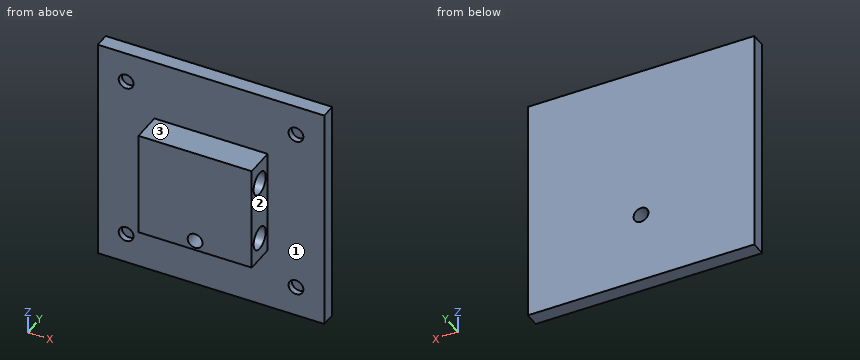
Autodesk Inventor part; units mm, degrees
ref_plane "YZ Plane" through (0, 0, 0) normal (1, 0, 0) x (0, 1, 0)
ref_plane "XZ Plane" through (0, 0, 0) normal (0, 1, 0) x (-1, 0, 0)
ref_plane "XY Plane" through (0, 0, 0) normal (0, 0, 1) x (1, 0, 0)
sketch "Sketch1" plane through (0, 0, 0) normal (1, 0, 0) x (0, 1, 0)
  line L0 (0, 0) -> (10, 0)
  line L1 (10, 0) -> (10, -20)
  line L2 (10, -20) -> (0, -20)
  line L3 (0, -20) -> (0, 0)
  circle A0 centre (5, 0) radius 3.81
  circle A1 centre (5, -20) radius 3.81
  line L4 (10, 0) -> (0, 0)
  line L5 (0, 0) -> (0, 7.62)
  line L6 (0, 7.62) -> (10, 7.62)
  line L7 (10, 7.62) -> (10, 0)
  line L8 (0, -20) -> (10, -20)
  line L9 (10, -20) -> (10, -27.62)
  line L10 (10, -27.62) -> (0, -27.62)
  line L11 (0, -27.62) -> (0, -20)
  dimension "d0" = 10
  dimension "d1" = 20
  dimension "d2" = 7.62
  dimension "d3" = 7.62
  dimension "d4" = 10
  dimension "d5" = 7.62
  dimension "d7" = 7.62
extrude "Extrusion1" add sketch "Sketch1" along normal blind 38.1
extrude "Extrusion2" cut sketch "Sketch1" along normal blind 38.1 contours A0 L0 | L0 A0 | A1 L2 | L2 A1
sketch "Sketch2" plane through (0, 10, 7.62) normal (0, 1, 0) x (1, 0, 0)
  line L0 (57.15, -20.4851) -> (-19.05, -20.4851)
  line L1 (-19.05, -20.4851) -> (-19.05, 55.7149)
  line L2 (-19.05, 55.7149) -> (57.15, 55.7149)
  line L3 (57.15, 55.7149) -> (57.15, -20.4851)
  line L4 (57.15, -20.4851) -> (-19.05, 55.7149) construction
  line L5 (-19.05, -20.4851) -> (57.15, 55.7149) construction
  line L6 (0, 0) -> (38.1, 0)
  line L7 (0, 35.24) -> (38.1, 35.24)
  line L8 (-19.05, 17.6149) -> (4.7227, 17.6149)
  line L9 (57.15, 17.6149) -> (33.3773, 17.6149)
  circle A0 centre (4.7227, 17.6149) radius 2.5
  circle A1 centre (33.3773, 17.6149) radius 2.5
  line L10 (19.05, 55.7149) -> (19.05, 31.9422)
  circle A2 centre (19.05, 31.9422) radius 2.5
  point P0 (0, 7.62)
  point P1 (19.05, 17.6149)
  dimension "d12" = 17.6149
  dimension "d13" = 17.6251
  dimension "d14" = 35.24
  dimension "d15" = 76.2
  dimension "d16" = 76.2
  dimension "d17" = 19.05
  dimension "d32" = 23.7727
  dimension "d33" = 23.7727
  dimension "d34" = 5
  dimension "d35" = 5
  dimension "d38" = 23.7727
  dimension "d39" = 5
extrude "Extrusion3" add sketch "Sketch2" along normal blind 5 contours A1 | A2 | A0 | L0 L1 L2 L3
sketch "Sketch3" plane through (0, 10, 7.62) normal (0, -1, 0) x (1, 0, 0)
  line L0 (0, 0) -> (38.1, 0)
  line L1 (0, 0) -> (-19.05, 20.4851)
  line L2 (-19.05, 20.4851) -> (-19.05, -55.7149)
  line L3 (-19.05, -55.7149) -> (0, -35.2882)
  line L4 (57.15, -55.7149) -> (57.15, 20.4851)
  line L5 (57.15, -55.7149) -> (38.1, -35.2882)
  line L6 (38.1, 0) -> (57.15, 20.4851)
  circle A0 centre (47.625, -45.5015) radius 2.5
  circle A1 centre (47.625, 10.2425) radius 2.5
  circle A2 centre (-9.525, -45.5015) radius 2.5
  circle A3 centre (-9.525, 10.2425) radius 2.5
  point P0 (0, -7.62)
  dimension "d20" = 5
  dimension "d21" = 5
  dimension "d22" = 5
  dimension "d23" = 5
  dimension "d24" = 42.921
  dimension "d25" = 43.003
  dimension "d26" = 43.003
  dimension "d27" = 0
  dimension "d28" = 9.525
  dimension "d29" = 57.15
extrude "Extrusion4" cut sketch "Sketch3" against normal blind 2
extrude "Extrusion6" cut sketch "Sketch2" along normal mid plane 25.4 contours A2
thread "Thread1"
properties part number "plateform"
Verification items for the finished model (mm, model axes). Face numbers are marked on the shaded views. A direction names the side the tool comes from. Coordinates: 2 decimals unless noted, no trailing zeros. Order: outer loops, then holes, each group sorted by start corner. A loop starts at its lowest first (then second) coordinate and runs counter-clockwise, first axis right, second up. Notation, with made-up numbers: M 27.5,79.25 L 33.5,79.25 A22 ccw 33.5,114.25 Z; hole C -2.5,69 d11. An arc over 180 degrees is marked long. One line per item, written item: value. Start each with the question number.
Item 1: Sectioned sample at A-A (x = 19.05). Enter the section's corners in (y, z), then the cut area to 3 significant figures.
Item 2: Sectioned sample at B-B (z = 0). Enter the section's corners in (x, y).
Item 3: Access from +Z, -Z, +X, -X, +Y, -Y to the whole of each face (thin tool, end or side, straight path). Record for the marked faces 1, 2 and 3.
Item 4: Sectioned sample at C-C (x = 9). Enter the section's corners in (y, z), then the cut area to 3 significant figures.
Item 5: Scan lines: probe 1 along Z at (x, y) = (14, 5); probe 2 along X at (y, z) = (6.25, -24.5); probe 3 along Y at (x, z) = (20, -20). Record each from-to range of solid material in increasing order.
Item 6: Gauge pin test, flat ends, axial feed: pin 1 (2.5 mm diameter, centred on x = -10.5, z = 17.5, fed in from -Y); pin 2 (6 mm diameter, centred on x = 47.62, z = 17.86, fed in from -Y); pin 3 (3 mm diameter, centred on x = 25, y = 4, fed in from -Z). Record the tip position at first contact, or that the pin passes through.
Item 7: Sectioned sample at D-D (y = 5). Enter the section's corners in (x, z), then the cut area to 3 significant figures.
Conclusion:
1. outline: M 0,-27.62 L 10,-27.62 L 10,-48.09 L 15,-48.09 L 15,-26.82 L 0,-26.82 Z; M 0,-21.82 L 1.65,-21.82 A3.81 cw long 8.35,-21.82 L 15,-21.82 L 15,28.11 L 10,28.11 L 10,7.62 L 0,7.62 Z; hole C 5,0 d7.62
1. area: 577 mm^2
2. outline: M -19.05,10 L 0,10 L 0,8.81 L 38.1,8.81 L 38.1,10 L 57.15,10 L 57.15,15 L -19.05,15 Z; M 0,0 L 38.1,0 L 38.1,1.19 L 0,1.19 Z
3. face 1: -Y
3. face 2: +Z, -Z, +X, -Y
3. face 3: +Z, +X, -X, -Y
4. outline: M 0,-27.62 L 10,-27.62 L 10,-48.09 L 15,-48.09 L 15,28.11 L 10,28.11 L 10,7.62 L 0,7.62 Z; hole C 5,-20 d7.62; hole C 5,0 d7.62
4. area: 642 mm^2
5. probe 1: z = -27.62 to -23.81, -16.19 to -3.81, 3.81 to 7.62
5. probe 2: x = 0 to 16.56, 21.54 to 38.1
5. probe 3: y = 0 to 1.19, 8.81 to 15
6. pin 1: stops at y = 12
6. pin 2: stops at y = 10
6. pin 3: stops at z = -27.62
7. outline: M 0,-27.62 L 38.1,-27.62 L 38.1,-23.81 L 21.5,-23.81 A2.5 cw long 16.6,-23.81 L 0,-23.81 Z; M 0,-16.19 L 38.1,-16.19 L 38.1,-3.81 L 0,-3.81 Z; M 0,3.81 L 38.1,3.81 L 38.1,7.62 L 0,7.62 Z
7. area: 750 mm^2
